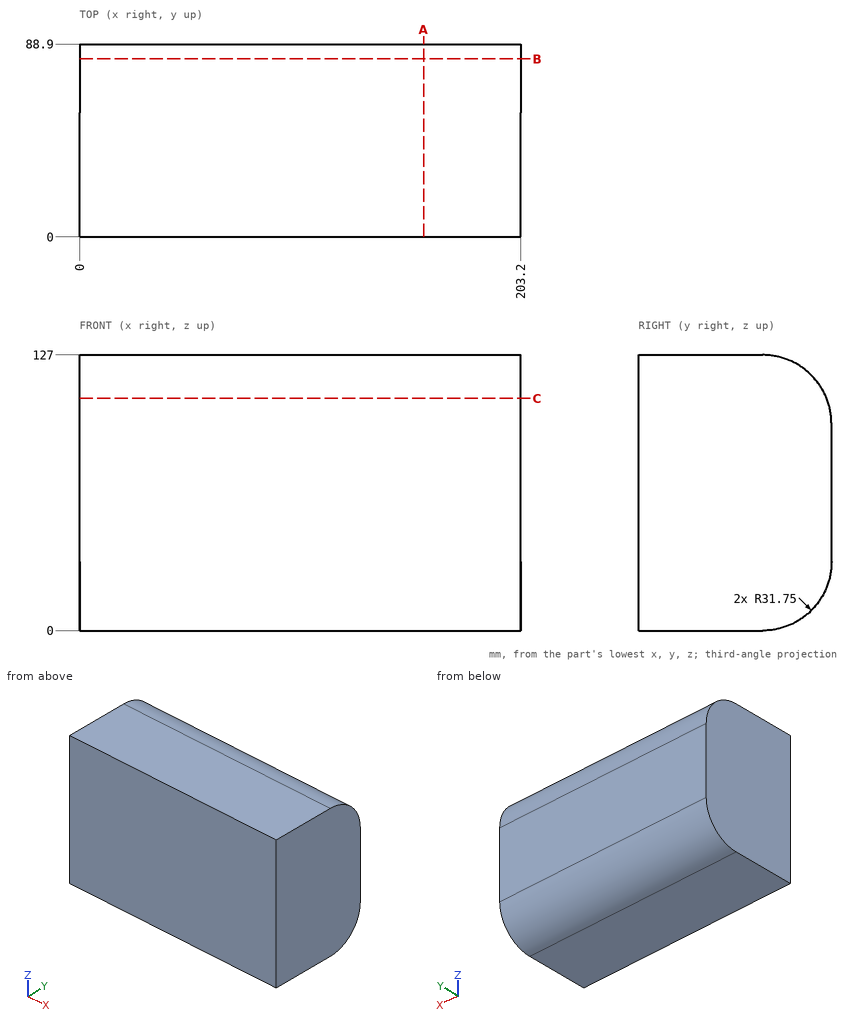
Job drawing, mm, ordinate dimensions from the low corner. One solid piece. Give positions to 0.01 mm unless a question says otherwise; leave off trailing zeros. Loops run counter-clockwise (first coordinate to the right, second up) from the corner with the lowest first, then second, coordinate; pieces in that order, holes last. Notation, with made-up numbers: (62.5, 26) -> (78.5, 26) arc R15 ccw to (78.5, 44) -> close; hole circle Ø9 at (-38, 88). An arc over 180 degrees is marked (long way). Write each question's results on one line, items separated by ' | '.
(1) Flat gauge pins, fed straight in: pin 1 Ø12 at (x, z) = (148, 113) entering from +Y; pin 2 Ø3 at (y, z) = (29, 84) entering from -X. Where does each tip first touch, or does it go through?
Geometry results:
pin 1: stops at y = 86.65 | pin 2: stops at x = 0
(2) Cut at B-B on y = 82. List the corners of the cut face in (x, z).
Geometry results:
outline: (0, 11.99) -> (203.2, 11.99) -> (203.2, 115.01) -> (0, 115.01) -> close
(3) Cut at C-C on z = 107. List the corners of the cut face in (x, y), and give its area (3 significant figures).
Geometry results:
outline: (0, 0) -> (203.2, 0) -> (203.2, 86.65) -> (0, 86.65) -> close | area: 17,600 mm²
(4) Probe line 1 along Y through (x, z) = (150.5, 95.5); line 2 along Z through (x, y) = (29.5, 85); line 3 along Y through (x, z) = (184, 5). List the from-to ranges inside material, lowest first.
Geometry results:
line 1: y = 0 to 88.9 | line 2: z = 16.5 to 110.5 | line 3: y = 0 to 74.25
(5) Cut at A-A on x = 158.5. List the corners of the cut face in (y, z).
Geometry results:
outline: (0, 0) -> (57.15, 0) arc R31.75 ccw to (88.9, 31.75) -> (88.9, 95.25) arc R31.75 ccw to (57.15, 127) -> (0, 127) -> close
